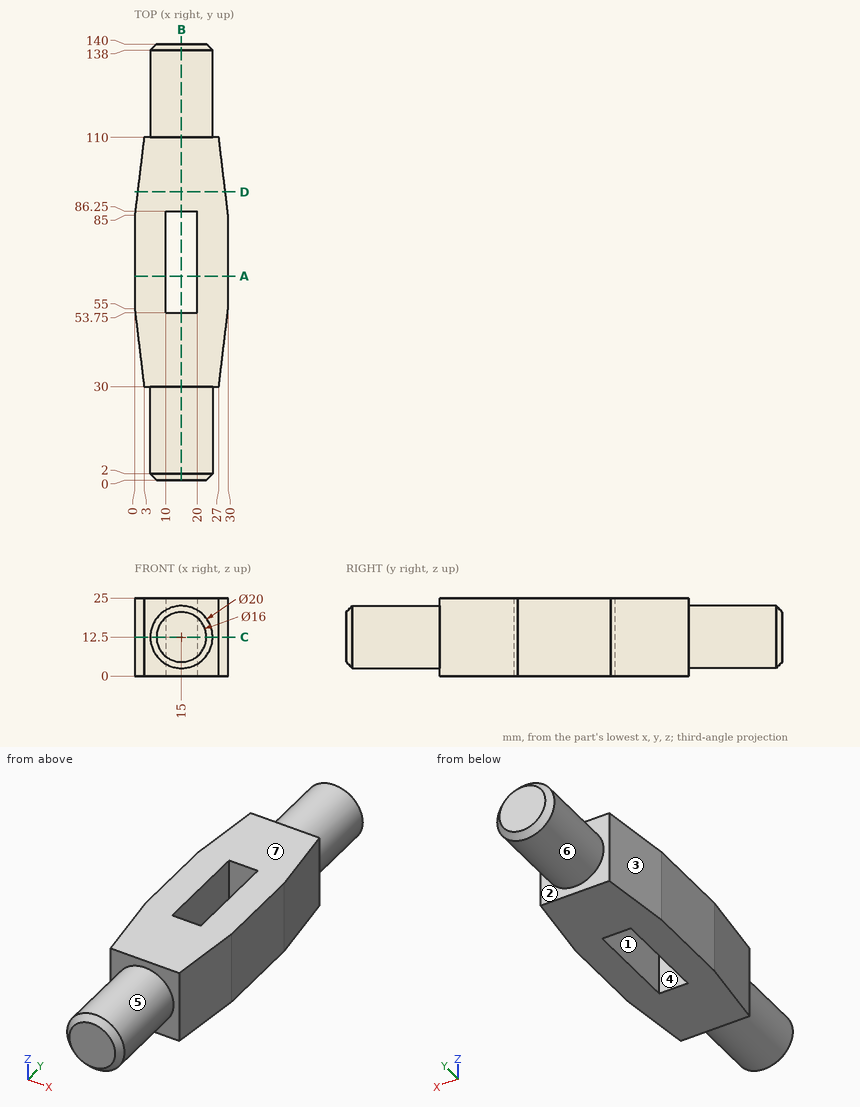
The drawing under review shows one solid part. Ordinate dimensions are in mm from its lowest x, y, z. A direction names the side the tool comes from. Coordinates: 2 decimals unless noted, no trailing zeros. Write each loop counter-clockwise with the first axis right and the second up, starting at its lowest first coordinate (ties: lowest second). Pieces come first, ordered by that corner, then holes. Notation, with made-up numbers: (37.25, -27) -> (44.25, -27) arc R28 ccw to (44.25, 10) -> close; hole circle Ø2 at (75, 62.25). An arc over 180 degrees is marked (long way). One line per item, written item: value. Start each with the question number.
Q1. The part is to be moulded in two halves that separate along X. For the marked faces 1, 2 and 3, say which applies: +X half, -X half, draft (parallel to the pull), parting line (faces both ways), or undercut.
Q2. Add section A-A, the plane y = 65.5. Give the boundary of the cut face in (x, z), then the cut area to 3 significant figures.
Q3. Add section B-B, the plane x = 15. Give the boundary of the cut face in (y, z).
Q4. Clearance check with flat-ended pins moving along their axes: P1, Ø1, axis at y = 122.5, z = 12, coming from the +X side; P2, Ø5, axis at y = 26, z = 4.5, coming from the +X side; P3, Ø1.5, axis at y = 42, z = 6, coming from the +X side. State where each tip first meets the part, or that it passes through.
Q5. Add section C-C, the plane z = 12.5. Give the boundary of the cut face in (x, y), then the cut area to 3 significant figures.
Q6. To check wall thickness, follow probe 1 along X at (y, z) = (84, 16); probe 2 along Y at (x, z) = (11, 3.25); probe 3 along Y at (x, z) = (15.25, 17.5). State the ranges of each line that lie inside material, in increasing order.
Q7. For the marked faces 4, 5, 6 and 7, list the 3-axis set-ups (+Z, -Z, +X, -X, +Y, -Y) from which the entire face can be reached by the end or side of a thin tool; tool diameter is ignored.
Q8. Add section D-D, the plane y = 92.5. Give the boundary of the cut face in (x, z), then the cut area to 3 significant figures.
Response:
1. face 1: undercut
1. face 2: draft
1. face 3: -X half
2. outline: (0, 0) -> (10, 0) -> (10, 25) -> (0, 25) -> close; (20, 0) -> (30, 0) -> (30, 25) -> (20, 25) -> close
2. area: 500 mm²
3. outline: (0, 4.5) -> (2, 2.5) -> (30, 2.5) -> (30, 0) -> (53.75, 0) -> (53.75, 25) -> (30, 25) -> (30, 22.5) -> (2, 22.5) -> (0, 20.5) -> close; (86.25, 0) -> (110, 0) -> (110, 2.5) -> (138, 2.5) -> (140, 4.5) -> (140, 20.5) -> (138, 22.5) -> (110, 22.5) -> (110, 25) -> (86.25, 25) -> close
4. P1: x = 25
4. P2: x = 23.35
4. P3: x = 28.53
5. outline: (0, 55) -> (3, 30) -> (5, 30) -> (5, 2) -> (7, 0) -> (23, 0) -> (25, 2) -> (25, 30) -> (27, 30) -> (30, 55) -> (30, 85) -> (27, 110) -> (25, 110) -> (25, 138) -> (23, 140) -> (7, 140) -> (5, 138) -> (5, 110) -> (3, 110) -> (0, 85) -> close; hole (10, 53.75) -> (20, 53.75) -> (20, 86.25) -> (10, 86.25) -> close
5. area: 3,120 mm²
6. probe 1: 0 to 10, 20 to 30
6. probe 2: 30 to 53.75, 86.25 to 110
6. probe 3: 0 to 53.75, 86.25 to 140
7. face 4: +Z, -Z
7. face 5: -Y
7. face 6: +Y
7. face 7: +Z, +X, -X, +Y, -Y
8. outline: (0.9, 0) -> (29.1, 0) -> (29.1, 25) -> (0.9, 25) -> close
8. area: 705 mm²
